```python
from build123d import *

# Parameters (mm, degrees)
SKETCH1_R           = 6
BOSS_EXTRUDE1_DEPTH = 59.25
SKETCH3_R           = 3
BOSS_EXTRUDE3_DEPTH = 7.5
BOSS_EXTRUDE4_START = 30
SKETCH2_R           = 3
BOSS_EXTRUDE4_DEPTH = 30


with BuildPart() as part:
    # Sketch1 → Boss-Extrude1 (new, symmetric)
    with BuildSketch(Plane.XY):
        Circle(SKETCH1_R)
    extrude(amount=BOSS_EXTRUDE1_DEPTH, both=True)

    # Sketch3 → Boss-Extrude3 (add)
    with BuildSketch(Plane(origin=(0, 0, -59.25), x_dir=(-1, 0, 0), z_dir=(0, 0, -1))):
        with Locations(Location((0, 0, 0), (0, 0, 180))):
            Circle(SKETCH3_R)
    extrude(amount=BOSS_EXTRUDE3_DEPTH)

    # Sketch2 → Boss-Extrude4 (add)
    with BuildSketch(Plane.XY.offset(59.25).offset(BOSS_EXTRUDE4_START)):
        Circle(SKETCH2_R)
    extrude(amount=-BOSS_EXTRUDE4_DEPTH)


solid = part.part
```
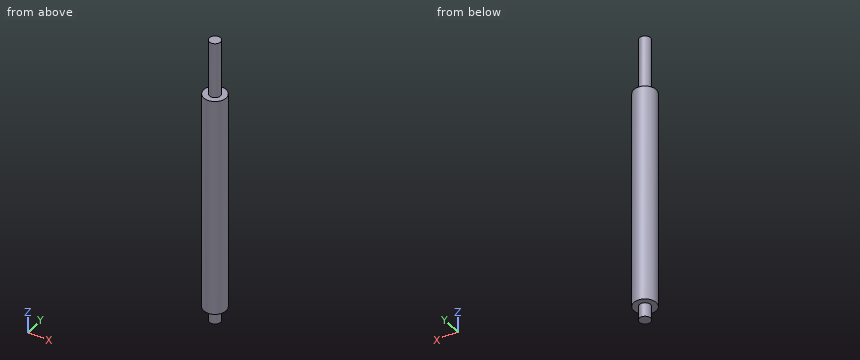
Model file for the job. Use its own axes, mm. Coordinates: 2 decimals unless noted, no trailing zeros. Order: outer loops, then holes, each group sorted by start corner. A loop starts at its lowest first (then second) coordinate and runs counter-clockwise, first axis right, second up. Notation, with made-up numbers: (80.25, 20.25) -> (102.25, 20.25) arc R23 ccw to (102.25, 34.25) -> close; hole circle Ø3 at (-37.5, -34.75). An arc over 180 degrees is marked (long way). Answer as a JSON object with one key per item and string values. Group by question number.
1) Cut at A-A, the plane x = 0. Write the cut outline in (y, z), then the cut area to 3 significant figures.
2) Cut at C-C, the plane z = -45.5. Write the cut outline in (x, y), then the cut area to 3 significant figures.
3) Drill centre lines: L1, parallel to X at y = -0.5, z = -31.5; L2, parallel to Z at x = -3.5, y = 4; L3, parallel to X at y = 5.25, z = 9. Where is each one in solid material? Low to high.
4) Flat gauge pins, fed straight in: pin 1 (1 mm diameter, centred on x = 1, z = -5, fed in from -Y); pin 2 (3 mm diameter, centred on x = -2, y = -3.5, fed in from -Z); pin 3 (4 mm diameter, centred on y = -3, z = 21.5, fed in from +X). Where does each tip first touch, or does it go through?
5) Cut at D-D, the plane z = 65.5. Write the cut outline in (x, y).
Check values:
{
 "1": {"outline": "(-6, -59.25) -> (-3, -59.25) -> (-3, -66.75) -> (3, -66.75) -> (3, -59.25) -> (6, -59.25) -> (6, 59.25) -> (3, 59.25) -> (3, 89.25) -> (-3, 89.25) -> (-3, 59.25) -> (-6, 59.25) -> close", "area": "1,650 mm²"},
 "2": {"outline": "circle Ø12 at (0, 0)", "area": "113 mm²"},
 "3": {"L1": "x = -5.98 to 5.98", "L2": "z = -59.25 to 59.25", "L3": "x = -2.9 to 2.9"},
 "4": {"pin 1": "stops at y = -5.98", "pin 2": "stops at z = -66.75", "pin 3": "stops at x = 5.92"},
 "5": {"outline": "circle Ø6 at (0, 0)"}
}
